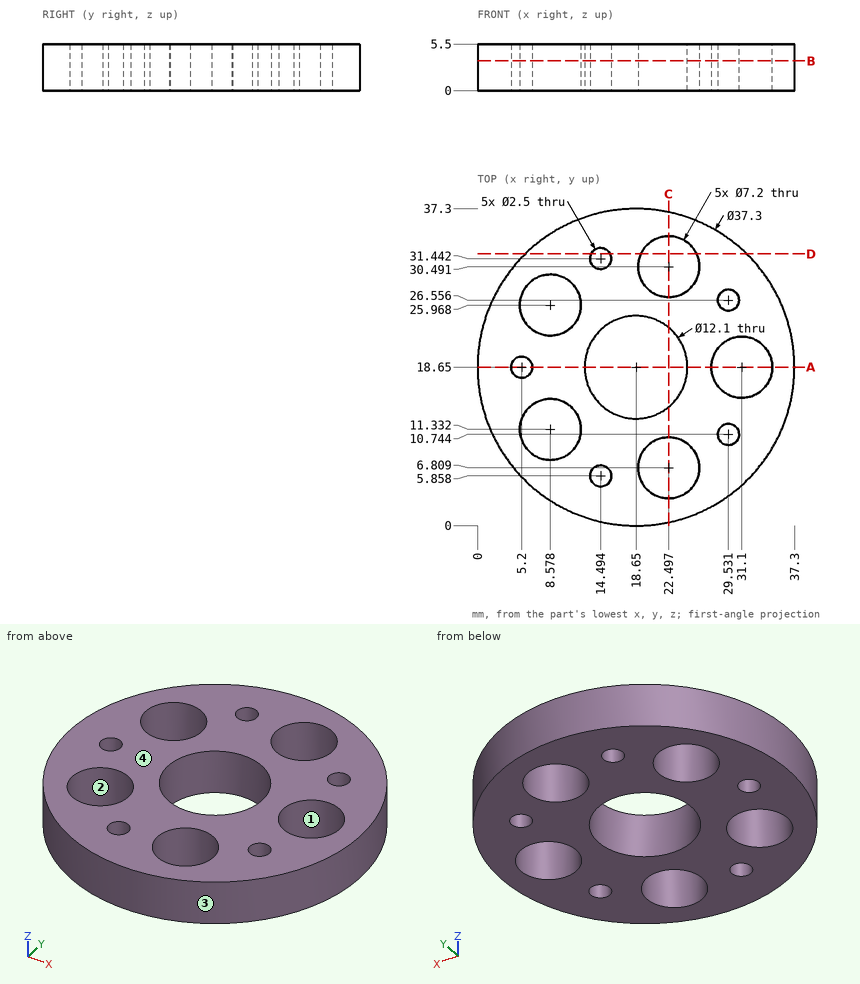
Design review of the part shown in the three views and the two pictorial views. Dimensions are in mm from the part's minimum x, y and z. Round coordinates to 2 decimals unless told otherwise and drop trailing zeros. Write each loop counter-clockwise with the first axis right and the second up, starting at its lowest first coordinate (ties: lowest second). Pieces come first, ordered by that corner, then holes. Notation, with made-up numbers: (80, 19.5) -> (85, 19.5) arc R12 cw to (85, 34.5) -> close; hole circle Ø7 at (53.5, 82.5). An arc over 180 degrees is marked (long way). One line per question, with ' | ' between items. Start each with the question number.
1) Add section A-A (y = 18.65). Write out the cut boundary in (x, z).
2) Add section D-D (y = 32). Write out the cut boundary in (x, z) (1 decimal), and give its area (3 significant figures).
3) Add section B-B (z = 3.5). Count the separate pieces of the cut face and the enclosed holes in it.
4) Add section C-C (x = 22.5). Write out the cut boundary in (y, z).
5) Wall thickness on line 1 along Y through (x, z) = (7, 3.65) (1 decimal); line 2 along Y through (x, z) = (18.65, 1.8); line 3 along X through (y, z) = (17, 4.15): over which ranges is each line inside the solid? List them lowest first.
6) Mouldability with a two-part tool opening along Y and no side actions: class the marked faces 1, 2, 3 and 4 as +Y half, -Y half, draft (parallel to the pull), parting line (faces both ways), or undercut.
7) For pin 1 Ø9.5 at (x, y) = (31.1, 18.65) entering from -Z; pin 2 Ø3 at (y, z) = (4, 2.5) entering from +X (1 decimal); pin 3 Ø1 at (x, z) = (20, 1) entering from -Y, all flat-tipped, find the tip position at first contact; note any pin that passes through.
Reported:
1) outline: (0, 0) -> (3.95, 0) -> (3.95, 5.5) -> (0, 5.5) -> close; (6.45, 0) -> (12.6, 0) -> (12.6, 5.5) -> (6.45, 5.5) -> close; (24.7, 0) -> (27.5, 0) -> (27.5, 5.5) -> (24.7, 5.5) -> close; (34.7, 0) -> (37.3, 0) -> (37.3, 5.5) -> (34.7, 5.5) -> close
2) outline: (5.6, 0) -> (13.4, 0) -> (13.4, 5.5) -> (5.6, 5.5) -> close; (15.6, 0) -> (19.2, 0) -> (19.2, 5.5) -> (15.6, 5.5) -> close; (25.8, 0) -> (31.7, 0) -> (31.7, 5.5) -> (25.8, 5.5) -> close | area: 95.0 mm²
3) separate pieces: 1 | enclosed holes: 11
4) outline: (0.4, 0) -> (3.21, 0) -> (3.21, 5.5) -> (0.4, 5.5) -> close; (10.41, 0) -> (13.98, 0) -> (13.98, 5.5) -> (10.41, 5.5) -> close; (23.32, 0) -> (26.89, 0) -> (26.89, 5.5) -> (23.32, 5.5) -> close; (34.09, 0) -> (36.9, 0) -> (36.9, 5.5) -> (34.09, 5.5) -> close
5) line 1: y = 4.1 to 8.1, 14.6 to 22.7, 29.2 to 33.2 | line 2: y = 0 to 12.6, 24.7 to 37.3 | line 3: x = 0.07 to 12.83, 24.47 to 27.9, 34.3 to 37.23
6) face 1: undercut | face 2: undercut | face 3: parting line | face 4: draft
7) pin 1: stops at z = 0 | pin 2: stops at x = 31.9 | pin 3: stops at y = 0.02
